```python
from build123d import *

# Parameters (mm, degrees)
SKETCH1_W           = 195
SKETCH1_H           = 195
SKETCH1_R           = 20
SKETCH1_RX          = 20.136316196
SKETCH1_RY          = 12.177676937
SKETCH1_W_2         = 32.002781641
SKETCH1_H_2         = 32.002781641
BOSS_EXTRUDE1_DEPTH = 10


with BuildPart() as part:
    # Sketch1 → Boss-Extrude1 (new body)
    with BuildSketch(Plane.XY):
        Rectangle(SKETCH1_W, SKETCH1_H)
        with Locations((-68.819541029, 68.819541029)):
            Circle(SKETCH1_R, mode=Mode.SUBTRACT)
        with Locations(Location((-68.819541029, -68.819541029), (0, 0, 45))):
            Ellipse(SKETCH1_RX, SKETCH1_RY, mode=Mode.SUBTRACT)
        Polygon((68.819541029, 44.07162726), (90.251863044, 81.193497914), (47.387219014, 81.193497914), align=None, mode=Mode.SUBTRACT)
        with Locations((68.81954103, -68.81954103)):
            Rectangle(SKETCH1_W_2, SKETCH1_H_2, mode=Mode.SUBTRACT)
    extrude(amount=BOSS_EXTRUDE1_DEPTH)


solid = part.part
```
Can you work these out from the model? Positions are in its coordinate system, mm. A direction names the side the tool comes from. Coordinates: 2 decimals unless noted, no trailing zeros. Write each loop counter-clockwise with the first axis right and the second up, starting at its lowest first coordinate (ties: lowest second). Pieces come first, ordered by that corner, then holes. Notation, with made-up numbers: M -24.75,79.25 L 24.25,79.25 A11 cw 24.25,100.25 Z; hole C 5.25,35 d4. An arc over 180 degrees is marked long. Write item = value, one per line. Start each with the question number.
Q1. If I drill on L1, parallel to Y at x = 66, z = 8.25; L2, parallel to X at y = -56.5, z = 6.5; L3, parallel to X at y = 59.5, z = 7.75, over which ranges is the centre line in solid material (lowest first)? Write a range as [from, to].
Q2. On a 3-axis mill with a long thin cutter (end or side, diameter ignored), from which of +Z, -Z, +X, -X, +Y, -Y can I reach the whole of each face in a straight line? I mean faces 4 (the face through (69, -84.821, 5)), 5 (the face through (97.5, -1, 5)). Say none if no direction works.
Q3. Thinking about a two-plate mould opening in Y: for faces 1 (the face through (69, -52.818, 5)), 2 (the face through (-1, 97.5, 5)), 3 (the face through (-97.5, -1, 5)), which applies, released by +Y, released by -Y, zero draft, split by the parting line, or undercut?
Q4. If we section it at C-C, the plane z = 8.5: State how many separate pieces and enclosed holes the cut face has, then the cut area to 3 significant figures.
Q5. If we section it at A-A, the plane y = 55: Write out the boundary of the cut face in (x, z).
Q6. If we section it at B-B, the plane x = 57: Write out the boundary of the cut face in (y, z).
Check sheet entries:
q1.L1 = [-97.5, -84.82], [-52.82, 48.96], [81.19, 97.5]
q1.L2 = [-97.5, -73], [-53.19, 52.82], [84.82, 97.5]
q1.L3 = [-97.5, -86.52], [-51.12, 59.91], [77.73, 97.5]
q2.face_4 = +Z, -Z
q2.face_5 = +Z, -Z, +X, +Y, -Y
q3.face_1 = undercut
q3.face_2 = released by +Y
q3.face_3 = zero draft
q4.separate_pieces = 1
q4.enclosed_holes = 4
q4.area = 34,200 mm²
q5.outline = M -97.5,0 L -83.28,0 L -83.28,10 L -97.5,10 Z; M -54.36,0 L 62.51,0 L 62.51,10 L -54.36,10 Z; M 75.13,0 L 97.5,0 L 97.5,10 L 75.13,10 Z
q6.outline = M -97.5,0 L -84.82,0 L -84.82,10 L -97.5,10 Z; M -52.82,0 L 64.54,0 L 64.54,10 L -52.82,10 Z; M 81.19,0 L 97.5,0 L 97.5,10 L 81.19,10 Z
